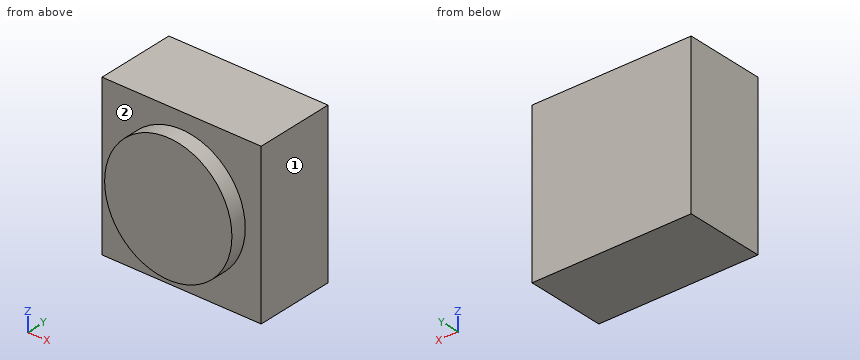
```python
from build123d import *

# Parameters (mm, degrees)
F0_W     = 12.7
F0_H     = 25.4
F1_DEPTH = 6.35
F2_DEPTH = 6.35
F3_R     = 10.16
F4_DEPTH = 2.54


with BuildPart() as f1:
    # F0 (on Front) → F1 (new body, symmetric)
    with BuildSketch(Plane.XZ):
        Rectangle(F0_W, F0_H)
    extrude(amount=F1_DEPTH, both=True)

    # F0 (on Front) → F2 (join, symmetric)
    with BuildSketch(Plane.XZ):
        with Locations((-12.7, 0)):
            Rectangle(F0_W, F0_H)
    extrude(amount=F2_DEPTH, both=True)

    # F3 (on face) → F4 (join)
    with BuildSketch(Plane.XZ.offset(6.35)):
        with Locations((-6.35, 0)):
            Circle(F3_R)
    extrude(amount=F4_DEPTH)


solid = f1.part
```
The model under review builds one solid part; all positions refer to its coordinate system, in mm. Face numbers are marked on the shaded views. A direction names the side the tool comes from. Give positions to 0.01 mm unless a question says otherwise; leave off trailing zeros. Write each loop counter-clockwise with the first axis right and the second up, starting at its lowest first coordinate (ties: lowest second). Pieces come first, ordered by that corner, then holes. Notation, with made-up numbers: (-3, -19.75) -> (9, -19.75) arc R30 cw to (9, 19.25) -> close; hole circle Ø5 at (25.25, 21.25). An arc over 180 degrees is marked (long way). Answer in a Markdown table with one row per item.
1) Clearance check with a flat-ended pin moving along its axis: P1, Ø1.5, axis at x = -9, y = -7.5, coming from the +Z side. State where the tip first meets the part, or that it passes through.
Worked answers:
| item | result |
|---|---|
| P1 | z = 9.98 |
2) Add section B-B on x = 2.75. State the section outline as (y, z) points, plus the area to 3 significant figures.
Worked answers:
| item | result |
|---|---|
| outline | (-8.89, -4.52) -> (-6.35, -4.52) -> (-6.35, -12.7) -> (6.35, -12.7) -> (6.35, 12.7) -> (-6.35, 12.7) -> (-6.35, 4.52) -> (-8.89, 4.52) -> close |
| area | 346 mm² |
3) Add section A-A on z = 0. State the section outline as (x, y) points.
Worked answers:
| item | result |
|---|---|
| outline | (-19.05, -6.35) -> (-16.51, -6.35) -> (-16.51, -8.89) -> (3.81, -8.89) -> (3.81, -6.35) -> (6.35, -6.35) -> (6.35, 6.35) -> (-19.05, 6.35) -> close |
4) For L1, parallel to Y at x = -15.75, z = 11.25; L2, parallel to X at y = -8.5, z = -2, list the stretches that pass through material, from the lowest coordinate up. Write a range as [from, to].
Worked answers:
| item | result |
|---|---|
| L1 | [-6.35, 6.35] |
| L2 | [-16.31, 3.61] |
5) Tool access review of the marked faces 1 and 2: name each direction out of +Z, -Z, +X, -X, +Y, -Y from which nothing blocks a thin tool from reaching the whole face with its end or side.
Worked answers:
| item | result |
|---|---|
| face 1 | +Z, -Z, +X, +Y, -Y |
| face 2 | -Y |
